Can you work these out from the model? Positions are in its coordinate system, mm. A direction names the side the tool comes from. Round coordinates to 2 decimals unless told otherwise and drop trailing zeros. Write each loop counter-clockwise with the first axis right and the second up, starting at its lowest first coordinate (ties: lowest second). Pieces come first, ordered by that corner, then holes. Notation, with made-up numbers: M -31.75,76.25 L 24.25,76.25 A14 ccw 24.25,81.25 Z; hole C 63,46.25 d3. An arc over 180 degrees is marked long. Answer in a Markdown table with one row per item. Add a question column.
(1) For faces 1 (the face through (-0.794, -8, -2)), 2 (the face through (0.794, -8, -2)), 3 (the face through (-2, -8, 0.794)), 4 (the face through (0.794, -8, 2)), which set-ups out of +Z, -Z, +X, -X, +Y, -Y let a thin tool reach every point of the face, with its end or its side?
(2) Suppose I cut it at A-A, the plane y = -8.75. Write out the boundary of the cut face in (x, z).
(3) Suppose I cut it at B-B, the plane x = -1. Write out the boundary of the cut face in (y, z) (3 decimals).
(4) Suppose I cut it at C-C, the plane z = -1.55. Write out the boundary of the cut face in (x, y) (3 decimals), then the cut area to 3 significant figures.
(5) I'm going to push flat-ended pins straight in: pin 1 (1.7 mm diameter, centred on y = -12, z = -2, fed in from +X); pin 2 (0.5 mm diameter, centred on y = -10.5, z = -1, fed in from -X); pin 3 (0.5 mm diameter, centred on x = 1.5, y = -10, fed in from -Z); pin 4 (0.8 mm diameter, centred on y = -7, z = 2, fed in from -X). Where does each tip first touch, or does it pass through?
(6) If I drill on probe 1 along X at (y, z) = (-3, -2.1), over which ranges is the centre line in solid material (lowest first)?
from build123d import *

# Parameters (mm, degrees)
F0_W     = 1.5875
F0_H     = 1.5875
F1_DEPTH = 15.875


with BuildPart() as f1:
    # F0 (on Front) → F1 (new body)
    with BuildSketch(Plane.XZ):
        with Locations((-1.5875, 0)):
            Rectangle(F0_W, F0_H)
        with Locations((0, 1.5875)):
            Rectangle(F0_W, F0_H)
        Rectangle(F0_W, F0_H)
        with Locations((1.5875, 0)):
            Rectangle(F0_W, F0_H)
        with Locations((0, -1.5875)):
            Rectangle(F0_W, F0_H)
    extrude(amount=F1_DEPTH)


solid = f1.part
Calculated:
| question | item | result |
|---|---|---|
| 1 | face 1 | -Z, -X, +Y, -Y |
| 1 | face 2 | -Z, +X, +Y, -Y |
| 1 | face 3 | +Z, -X, +Y, -Y |
| 1 | face 4 | +Z, +X, +Y, -Y |
| 2 | outline | M -2.38,-0.79 L -0.79,-0.79 L -0.79,-2.38 L 0.79,-2.38 L 0.79,-0.79 L 2.38,-0.79 L 2.38,0.79 L 0.79,0.79 L 0.79,2.38 L -0.79,2.38 L -0.79,0.79 L -2.38,0.79 Z |
| 3 | outline | M -15.875,-0.794 L 0,-0.794 L 0,0.794 L -15.875,0.794 Z |
| 4 | outline | M -0.794,-15.875 L 0.794,-15.875 L 0.794,0 L -0.794,0 Z |
| 4 | area | 25.2 mm² |
| 5 | pin 1 | x = 0.79 |
| 5 | pin 2 | x = -2.38 |
| 5 | pin 3 | z = -0.79 |
| 5 | pin 4 | x = -0.79 |
| 6 | probe 1 | -0.79 to 0.79 |
